Geometry check sheet. Reference: the model listing, model coordinates, mm. Coordinates: 2 decimals unless noted, no trailing zeros. Write each loop counter-clockwise with the first axis right and the second up, starting at its lowest first coordinate (ties: lowest second). Pieces come first, ordered by that corner, then holes. Notation, with made-up numbers: (25.25, 87.25) -> (56.25, 87.25) arc R27 cw to (56.25, 126.25) -> close; hole circle Ø1 at (-30.75, 62). An arc over 180 degrees is marked (long way). Answer in a Markdown table with one row per item. Add a question column.
Q1. Section check D-D, the plane z = 8. Record the boundary of the cut face in (x, y), and give its area (3 significant figures).
Q2. Section check C-C, the plane y = -1.75. Record the boundary of the cut face in (x, z).
Q3. Gauge pin test, flat ends, axial feed: P1, Ø8, axis at x = 23.06, z = 12.7, coming from the +Y side; P2, Ø1.9, axis at y = -1.5, z = 15.5, coming from the +X side. Record the tip position at first contact, or that the pin passes through.
Q4. Section check B-B, the plane x = 4. Record the boundary of the cut face in (y, z).
Q5. Release check for a two-part mould opening along X. For faces 1 (the face through (37.377, -8.634, 15.168)), 2 (the face through (11.049, -2, 13)), 3 (the face through (30, -6.286, 13)) record: pulls with the +X half, pulls with the -X half, needs draft (parallel to the pull), parting line crosses it, or undercut.
Q6. Section check A-A, the plane z = 13.75. Record the boundary of the cut face in (x, y), and give its area (3 significant figures).
Q7. Thickness scan on line 1 (X direction, y = 5.5, z = 8.25); line 2 (X direction, y = 4.5, z = 24.5); line 3 (Y direction, x = 43, z = 12.5). Record the ranges inside material, lowest first.
```python
from build123d import *

# Parameters (mm, degrees)
SKETCH1_R           = 6.35
BOSS_EXTRUDE1_DEPTH = 25.4
FILLET1_R           = 2.54
SKETCH2_R           = 2.4892
CUT_EXTRUDE1_DEPTH  = 5.7625


with BuildPart() as part:
    # Sketch1 → Boss-Extrude1 (new body)
    with BuildSketch(Plane.XY):
        with BuildLine():
            Line((11.049, -6.2865), (11.049, 0))
            ThreePointArc((11.049, 0), (-7.812822825, 7.812822825), (0, -11.049))
            Line((0, -11.049), (45.91627088, -11.049))
            Line((45.91627088, -11.049), (45.91627088, -6.2865))
            Line((45.91627088, -6.2865), (11.049, -6.2865))
        make_face()
        with Locations((0, 0.127)):
            Circle(SKETCH1_R, mode=Mode.SUBTRACT)
    extrude(amount=BOSS_EXTRUDE1_DEPTH)

    # Fillet1
    fillet1_edges = [part.edges().sort_by_distance(p)[0] for p in [
        (11.049, -6.2865, 12.7),
    ]]
    fillet(fillet1_edges, radius=FILLET1_R)

    # Sketch2 → Cut-Extrude1 (cut, through all)
    with BuildSketch(Plane(origin=(0, -6.2865, 0), x_dir=(1, 0, 0), z_dir=(0, 1, 0))):
        with Locations(Location((37.052858889, -12.7, 0), (0, 0, 180))):  # turned: the seam where the file's is
            Circle(SKETCH2_R)
        with Locations(Location((23.063244992, -12.7, 0), (0, 0, 180))):  # turned: the seam where the file's is
            Circle(SKETCH2_R)
    extrude(amount=-CUT_EXTRUDE1_DEPTH, mode=Mode.SUBTRACT)


solid = part.part
```
Calculated:
| question | item | result |
|---|---|---|
| 1 | outline | (0, -11.05) -> (45.92, -11.05) -> (45.92, -6.29) -> (13.59, -6.29) arc R2.54 cw to (11.05, -3.75) -> (11.05, 0) arc R11.05 ccw (long way) to start; hole circle Ø12.7 at (0, 0.13) |
| 1 | area | 450 mm² |
| 2 | outline | (-10.91, 0) -> (-6.07, 0) -> (-6.07, 25.4) -> (-10.91, 25.4) -> close; (6.07, 0) -> (11.05, 0) -> (11.05, 25.4) -> (6.07, 25.4) -> close |
| 3 | P1 | stops at y = -6.29 |
| 3 | P2 | stops at x = 11.05 |
| 4 | outline | (-11.05, 0) -> (-4.8, 0) -> (-4.8, 25.4) -> (-11.05, 25.4) -> close; (5.06, 0) -> (10.3, 0) -> (10.3, 25.4) -> (5.06, 25.4) -> close |
| 5 | face 1 | undercut |
| 5 | face 2 | pulls with the +X half |
| 5 | face 3 | needs draft |
| 6 | outline | (0, -11.05) -> (20.81, -11.05) -> (20.81, -6.29) -> (13.59, -6.29) arc R2.54 cw to (11.05, -3.75) -> (11.05, 0) arc R11.05 ccw (long way) to start; (25.32, -11.05) -> (34.8, -11.05) -> (34.8, -6.29) -> (25.32, -6.29) -> close; (39.31, -11.05) -> (45.92, -11.05) -> (45.92, -6.29) -> (39.31, -6.29) -> close; hole circle Ø12.7 at (0, 0.13) |
| 6 | area | 407 mm² |
| 7 | line 1 | x = -9.58 to -3.38, 3.38 to 9.58 |
| 7 | line 2 | x = -10.09 to -4.6, 4.6 to 10.09 |
| 7 | line 3 | y = -11.05 to -6.29 |
